Could you check a few things on this model? Use its own coordinates, in mm. Coordinates: 2 decimals unless noted, no trailing zeros. Order: outer loops, then holes, each group sorted by start corner. A loop starts at its lowest first (then second) coordinate and runs counter-clockwise, first axis right, second up. Notation, with made-up numbers: (74, -8.5) -> (123, -8.5) arc R36 ccw to (123, 26.5) -> close; hole circle Ø10 at (64, 21). An arc over 180 degrees is marked (long way). Put each result on its own line as item: value. Start each with the question number.
Q1. If we section it at B-B (z = 0.35): Please give me the cut outline in (x, y), and give its area (3 significant figures).
Q2. If we section it at A-A (x = 23): Please give me the cut outline in (y, z), and give its area (3 significant figures).
Q3. Will this pin go through, and if not, where does the flat tip stop? pin 1 (4 mm diameter, centred on x = 7.5, y = 0, fed in from -Z).
Q4. If we section it at C-C (y = -3): Please give me the cut outline in (x, z), and give its area (3 significant figures).
Q5. If we section it at D-D (y = 0): Please give me the cut outline in (x, z).
Q6. Please list where these lines run through material, in increasing order: line 1 along Y through (x, z) = (0, 0.85); line 2 along X through (y, z) = (-2.25, 0.75); line 3 along X through (y, z) = (-3.5, 0.9).
from build123d import *

# Parameters (mm, degrees)
SKETCH1_R           = 1
BOSS_EXTRUDE1_DEPTH = 1.5


with BuildPart() as part:
    # Sketch1 → Boss-Extrude1 (new body)
    with BuildSketch(Plane.XY):
        with BuildLine():
            ThreePointArc((1.477428659, 3.717150059), (-3.481097701, -1.970268712), (3.947365166, -0.646767534))
            ThreePointArc((3.947365166, -0.646767534), (11.5, 1), (19.052634834, -0.646767534))
            ThreePointArc((19.052634834, -0.646767534), (26.481097701, -1.970268712), (21.522571341, 3.717150059))
            ThreePointArc((21.522571341, 3.717150059), (11.5, 6), (1.477428659, 3.717150059))
        make_face()
        Circle(SKETCH1_R, mode=Mode.SUBTRACT)
        with Locations((23, 0)):
            Circle(SKETCH1_R, mode=Mode.SUBTRACT)
    extrude(amount=BOSS_EXTRUDE1_DEPTH)


solid = part.part
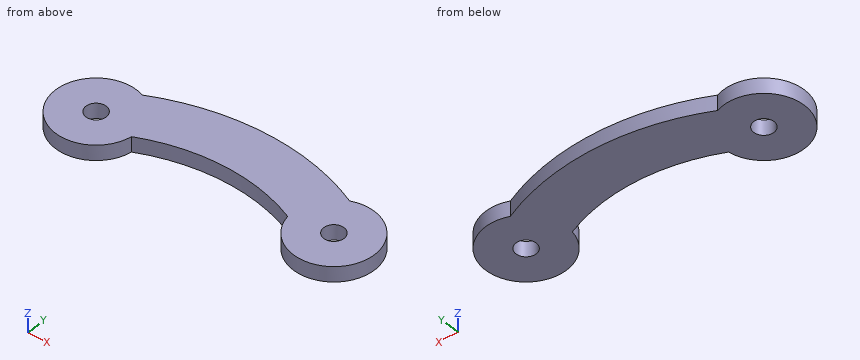
The answers:
1. outline: (1.48, 3.72) arc R4 ccw (long way) to (3.95, -0.65) arc R18.14 cw to (19.05, -0.65) arc R4 ccw (long way) to (21.52, 3.72) arc R23.14 ccw to start; hole circle Ø2 at (0, 0); hole circle Ø2 at (23, 0)
1. area: 179 mm^2
2. outline: (-4, 0) -> (-1, 0) -> (-1, 1.5) -> (-4, 1.5) -> close; (1, 0) -> (4, 0) -> (4, 1.5) -> (1, 1.5) -> close
2. area: 9.00 mm^2
3. pin 1: z = 0
4. outline: (-2.65, 0) -> (2.65, 0) -> (2.65, 1.5) -> (-2.65, 1.5) -> close; (20.35, 0) -> (25.65, 0) -> (25.65, 1.5) -> (20.35, 1.5) -> close
4. area: 15.9 mm^2
5. outline: (-4, 0) -> (-1, 0) -> (-1, 1.5) -> (-4, 1.5) -> close; (1, 0) -> (5.56, 0) -> (5.56, 1.5) -> (1, 1.5) -> close; (17.44, 0) -> (22, 0) -> (22, 1.5) -> (17.44, 1.5) -> close; (24, 0) -> (27, 0) -> (27, 1.5) -> (24, 1.5) -> close
6. line 1: -4 to -1, 1 to 4
6. line 2: -3.31 to 3.31, 19.69 to 26.31
6. line 3: -1.94 to 1.94, 21.06 to 24.94
